Source: CAD feature listing. Evaluate the final solid. Frame: model axes, mm. A direction names the side the tool comes from. Coordinates: 2 decimals unless noted, no trailing zeros. Write each loop counter-clockwise with the first axis right and the second up, starting at its lowest first coordinate (ties: lowest second). Pieces come first, ordered by that corner, then holes. Notation, with made-up numbers: (14, 89.5) - (58, 89.5) arc R25 cw to (58, 116.5) - close; hole circle Ø10 at (-2.75, 52.25). An arc over 180 degrees is marked (long way). One line per question, with ' | ' between items. Start each with the question number.
Q1. Line query: line 1 (Z direction, x = 123, y = 38); line 2 (Z direction, x = 12, y = 29); line 3 (Z direction, x = 68, y = 39). Output: solid intervals per line, ascending.
Q2. Access query for faces 5 (the face through (83.067, 19.855, -9.097)), 6 (the face through (39.74, 19.86, -22.31)), 7 (the face through (81.733, 20.404, -8.147)), 8 (the face through (15, 20, 0)), 9 (the face through (76.233, 20, -25)). Directions: +Z, -Z, +X, -X, +Y, -Y. A direction counts if a zero-diameter tool reaches every point of the face in a straight line with its end or side. Return the directions, or none.
Q3. Cut plane B-B, the plane y = 21.5. Give the number of separate pieces and of enclosed holes in the cut face, plus the area to 3 significant figures.
Q4. Contact query for flat-ended pins moving along their axis: P1, Ø8.5, axis at x = 37, z = -17.5, coming from the -Y side; P2, Ø6, axis at x = 82, y = 29.5, coming from the -Z side; P3, Ø6, axis at x = 154.5, y = 28, coming from the -Z side; P4, Ø2.5, axis at y = 17, z = -24, coming from the -X side. Output: stop coordinate, or through.
Q5. Cut plane A-A, the plane z = -11.25. Return loops of the section in (x, y).
Q6. Draft query along Z for faces 1 (the face through (82, 2.509, -16)), 2 (the face through (146.05, 21, -7)), 3 (the face through (125, 5, -6.615)), 4 (the face through (122, 34, -3.615)). Return one class per face: +Z half, -Z half, draft (parallel to the pull), parting line (faces both ways), or undercut.
```python
from build123d import *

# Parameters (mm, degrees)
BASE_FLANGE1_DEPTH  = 41
SKETCH2_W           = 42
SKETCH2_H           = 20
CUT_EXTRUDE1_DEPTH  = 10
BOSS_EXTRUDE1_DEPTH = 6
SKETCH5_R           = 1
CUT_EXTRUDE3_DEPTH  = 165.132308696
BOSS_EXTRUDE2_DEPTH = 41
SKETCH7_W           = 32.001348433
SKETCH7_H           = 33.78132576
CUT_EXTRUDE4_DEPTH  = 7
CUT_EXTRUDE5_START  = 2.509016302
CUT_EXTRUDE5_DEPTH  = 35.18539121
CUT_EXTRUDE6_START  = -3
CUT_EXTRUDE6_DEPTH  = 3


# Read off the part's stored shape, not the designer's step: Cut-Extrude5, Cut-Extrude6
# Sheet-metal steps are written as plain solids
with BuildPart() as part:
    # Sketch1 → Base-Flange1 (new body)
    with BuildSketch(Plane(origin=(0, 0, 0), x_dir=(1, 0, 0), z_dir=(0, 1, 0))):
        with BuildLine():
            Line((0, 0), (29.484227127, 0))
            ThreePointArc((29.484227127, 0), (29.90672353, 0.133212604), (30.176404712, 0.484667962))
            Line((30.176404712, 0.484667962), (38.681704054, 23.85278585))
            ThreePointArc((38.681704054, 23.85278585), (40.049733788, 25.635636911), (42.1929595, 26.311393382))
            Line((42.1929595, 26.311393382), (78.441184331, 26.311393382))
            ThreePointArc((78.441184331, 26.311393382), (80.843024514, 25.437195048), (82.121016981, 23.223647163))
            Line((82.121016981, 23.223647163), (84.942198964, 7.223929074))
            ThreePointArc((84.942198964, 7.223929074), (85.194131001, 6.787569985), (85.667608355, 6.615238322))
            Line((85.667608355, 6.615238322), (158.049527566, 6.615238322))
            Line((158.049527566, 6.615238322), (158.049527566, 3.615238322))
            Line((158.049527566, 3.615238322), (85.667608355, 3.615238322))
            ThreePointArc((85.667608355, 3.615238322), (83.265768172, 4.489436656), (81.987775705, 6.702984541))
            Line((81.987775705, 6.702984541), (79.166593722, 22.70270263))
            ThreePointArc((79.166593722, 22.70270263), (78.914661685, 23.139061719), (78.441184331, 23.311393382))
            Line((78.441184331, 23.311393382), (42.1929595, 23.311393382))
            ThreePointArc((42.1929595, 23.311393382), (41.770463097, 23.178180778), (41.500781916, 22.82672542))
            Line((41.500781916, 22.82672542), (32.995482574, -0.541392468))
            ThreePointArc((32.995482574, -0.541392468), (31.627452839, -2.324243529), (29.484227127, -3))
            Line((29.484227127, -3), (0, -3))
            Line((0, -3), (0, 0))
        make_face()
    extrude(amount=BASE_FLANGE1_DEPTH)

    # Sketch2 → Cut-Extrude1 (cut)
    with BuildSketch(Plane.XY.offset(-3.615238322)):
        with Locations((125.049527566, 20)):
            Rectangle(SKETCH2_W, SKETCH2_H)
    extrude(amount=-CUT_EXTRUDE1_DEPTH, mode=Mode.SUBTRACT)

    # Sketch3 → Boss-Extrude1 (add)
    with BuildSketch(Plane.XY.offset(-3.615238322)):
        Polygon((104.049527566, 30), (104.049527566, 41), (92.049527566, 41), (92.049527566, 0), (104.049527566, 0), (104.049527566, 10), align=None)
        Polygon((158.049527566, 0), (158.049527566, 41), (146.049527566, 41), (146.049527566, 30), (146.049527566, 10), (146.049527566, 0), align=None)
    extrude(amount=-BOSS_EXTRUDE1_DEPTH)

    # Sketch5 → Cut-Extrude3 (cut, through all)
    with BuildSketch(Plane(origin=(0, 0, -9.615238322), x_dir=(-1, 0, 0), z_dir=(0, 0, -1))):
        with Locations((-100.049527566, 25)):
            Circle(SKETCH5_R)
        with Locations((-100.049527566, 15)):
            Circle(SKETCH5_R)
        with Locations((-150.049527566, 15)):
            Circle(SKETCH5_R)
        with Locations((-150.049527566, 25)):
            Circle(SKETCH5_R)
    extrude(amount=-CUT_EXTRUDE3_DEPTH, mode=Mode.SUBTRACT)

    # Sketch6 → Boss-Extrude2 (add)
    with BuildSketch(Plane(origin=(0, 0, 0), x_dir=(-1, 0, 0), z_dir=(0, -1, 0))):
        with BuildLine():
            Line((-29.484227127, -3), (-75.34551542, -3))
            ThreePointArc((-75.34551542, -3), (-81.36937718, -1.03867544), (-85.667608355, 3.615238322))
            ThreePointArc((-85.667608355, 3.615238322), (-83.265768172, 4.489436656), (-81.987775705, 6.702984541))
            ThreePointArc((-81.987775705, 6.702984541), (-80.044156462, 1.965108483), (-75.315152978, 0))
            Line((-75.315152978, 0), (-29.484227127, 0))
            Line((-29.484227127, 0), (-29.484227127, -3))
        make_face()
    extrude(amount=-BOSS_EXTRUDE2_DEPTH)

    # Sketch7 → Cut-Extrude4 (cut)
    with BuildSketch(Plane.XY.offset(-23.311393382)):
        with Locations((60.232231791, 19.824471405)):
            Rectangle(SKETCH7_W, SKETCH7_H)
    extrude(amount=-CUT_EXTRUDE4_DEPTH, mode=Mode.SUBTRACT)

    # Cut-Extrude5 outline → Cut-Extrude5 (cut)
    with BuildSketch(Plane(origin=(0, 0, 0), x_dir=(1, 0, 0), z_dir=(0, 1, 0)).offset(CUT_EXTRUDE5_START)):
        Polygon((84.565358052, 9.361100086), (82.279466997, 22.325032469), (79.325043738, 21.804087936), (81.610934793, 8.840155553), align=None)
        Polygon((38.309494449, 22.830148366), (33.407161792, 9.361100086), (36.226239654, 8.335039656), (41.128572311, 21.804087936), align=None)
    extrude(amount=CUT_EXTRUDE5_DEPTH, mode=Mode.SUBTRACT)

    # Cut-Extrude6 outline → Cut-Extrude6 (cut)
    with BuildSketch(Plane.XY.offset(3).offset(CUT_EXTRUDE6_START)):
        with BuildLine():
            ThreePointArc((5.188265578, 0), (1.627560559, 1.417661865), (0, 4.887450335))
            Line((0, 4.887450335), (0, 0))
            Line((0, 0), (5.188265578, 0))
        make_face()
        with BuildLine():
            ThreePointArc((0, 35.818729295), (1.526422616, 39.473577384), (5.181270705, 41))
            Line((5.181270705, 41), (0, 41))
            Line((0, 41), (0, 35.818729295))
        make_face()
    extrude(amount=CUT_EXTRUDE6_DEPTH, mode=Mode.SUBTRACT)


solid = part.part
```
Reply:
1) line 1: z = -6.62 to -3.62 | line 2: z = 0 to 3 | line 3: z = -26.31 to -23.31, 0 to 3
2) face 5: none | face 6: -X | face 7: +Y, -Y | face 8: -Z, -X, +Y, -Y | face 9: -Z
3) separate pieces: 4 | enclosed holes: 0 | area: 505 mm^2
4) P1: stops at y = 0 | P2: stops at z = -26.27 | P3: stops at z = -9.62 | P4: stops at x = 38.31
5) outline: (34.09, 0) - (37.29, 0) - (37.29, 2.51) - (34.09, 2.51) - close; (34.09, 37.69) - (37.29, 37.69) - (37.29, 41) - (34.09, 41) - close; (81.19, 0) - (84.23, 0) - (84.23, 2.51) - (81.19, 2.51) - close; (81.19, 37.69) - (84.23, 37.69) - (84.23, 41) - (81.19, 41) - close
6) face 1: undercut | face 2: draft | face 3: -Z half | face 4: +Z half
